Geometry: final body of the model. Coordinates: model frame, mm. Face numbers are marked on the shaded views. A direction names the side the tool comes from. Round coordinates to 2 decimals unless told otherwise and drop trailing zeros. Order: outer loops, then holes, each group sorted by start corner. A loop starts at its lowest first (then second) coordinate and runs counter-clockwise, first axis right, second up. Notation, with made-up numbers: (-15, -20) - (26, -20) arc R27 ccw to (26, 17) - close; hole circle Ø1 at (20.5, -32.5). An arc over 180 degrees is marked (long way). Put each result on its own line as item: value. Start each with the question number.
(1) Pin query (flat end, axial travel): P1, Ø2, axis at y = 18, z = 11.5, coming from the +X side; P2, Ø3.5, axis at x = 7.5, z = 10, coming from the +Y side; P3, Ø6, axis at x = 29.5, z = 9, coming from the +Y side; P4, Ø8, axis at x = 5, y = 17.5, coming from the +Z side. Return the tip coordinate at first contact, or that it passes through.
(2) Section B-B (z = 4). Output: boundary loops of the cut face in (x, y), and give its area (3 significant figures).
(3) Section A-A (y = 12). Output: boundary loops of the cut face in (x, z), and give its area (3 significant figures).
(4) Pull-direction query (X, two-part tool) for the marked faces 5, 6 and 7; classes: released by +X, released by -X, zero draft, split by the parting line, or undercut.
(5) Access query for the marked faces 1, 2, 3 and 4. Directions: +Z, -Z, +X, -X, +Y, -Y. A direction counts if a zero-diameter tool reaches every point of the face in a straight line with its end or side. Return the directions, or none.
(6) Material intervals for L1, parallel to X at y = 5.5, z = 2.5; L2, parallel to Y at x = 36.5, z = 12.25; L3, parallel to Y at x = 27.5, z = 8, sorted ascending. Write a range as [from, to].
(7) Section D-D (y = 14.75). Output: boundary loops of the cut face in (x, z), and give its area (3 significant figures).
(8) Section C-C (x = 8). Output: boundary loops of the cut face in (y, z).
Autodesk Inventor part; units mm, degrees
ref_plane "YZ Plane" through (0, 0, 0) normal (1, 0, 0) x (0, 1, 0)
ref_plane "XZ Plane" through (0, 0, 0) normal (0, 1, 0) x (-1, 0, 0)
ref_plane "XY Plane" through (0, 0, 0) normal (0, 0, 1) x (1, 0, 0)
sketch "Sketch1" plane through (0, 0, 0) normal (0, 0, 1) x (1, 0, 0)
  line L0 (0, 0) -> (0, 3)
  line L1 (0, 3) -> (12, 3)
  line L2 (0, 0) -> (15, 0)
  line L3 (15, 0) -> (15, 13)
  line L4 (12, 3) -> (12, 13)
  line L5 (28, 13) -> (28, 0)
  line L6 (28, 0) -> (43, 0)
  line L7 (43, 0) -> (43, 3)
  line L8 (43, 3) -> (31, 3)
  line L9 (31, 3) -> (31, 13)
  arc A0 (28, 13) -> (15, 13) centre (21.5, 13) ccw
  arc A1 (31, 13) -> (12, 13) centre (21.5, 13) ccw
  dimension "d10" = 3
extrude "Extrusion1" add sketch "Sketch1" along normal blind 25.4
properties part number "SADDLE_CPY"
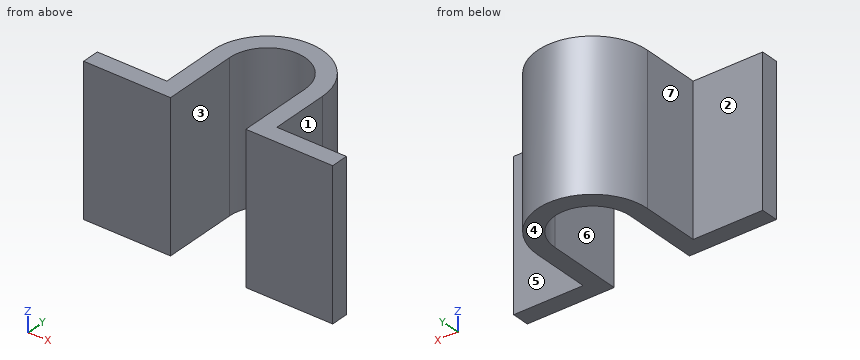
Checks:
1. P1: stops at x = 30.12
1. P2: stops at y = 3
1. P3: stops at y = 21.08
1. P4: passes through
2. outline: (0, 0) - (15, 0) - (15, 13) arc R6.5 cw to (28, 13) - (28, 0) - (43, 0) - (43, 3) - (31, 3) - (31, 13) arc R9.5 ccw to (12, 13) - (12, 3) - (0, 3) - close
2. area: 225 mm²
3. outline: (12, 0) - (15, 0) - (15, 25.4) - (12, 25.4) - close; (28, 0) - (31, 0) - (31, 25.4) - (28, 25.4) - close
3. area: 152 mm²
4. face 5: zero draft
4. face 6: undercut
4. face 7: released by -X
5. face 1: +Z, -Z, +X, +Y
5. face 2: +Z, -Z, -X, +Y
5. face 3: +Z, -Z, -Y
5. face 4: -Z, +X, -X, +Y, -Y
6. L1: x = [12, 15], [28, 31]
6. L2: y = [0, 3]
6. L3: y = [15.5, 20.37]
7. outline: (12.16, 0) - (15.24, 0) - (15.24, 25.4) - (12.16, 25.4) - close; (27.76, 0) - (30.84, 0) - (30.84, 25.4) - (27.76, 25.4) - close
7. area: 156 mm²
8. outline: (0, 0) - (3, 0) - (3, 25.4) - (0, 25.4) - close
